from build123d import *

# Parameters (mm, degrees)
SKETCH1_W           = 304.8
SKETCH1_H           = 89.8
SKETCH1_R           = 14.2875
SKETCH1_R_2         = 2.54
SKETCH1_R_3         = 17.145
BOSS_EXTRUDE1_DEPTH = 6.35
SKETCH2_W           = 114.9
SKETCH2_H           = 89.8
SKETCH2_R           = 2.54
SKETCH2_R_2         = 17.145
CUT_EXTRUDE1_DEPTH  = 10
SKETCH4_R           = 6.35
SKETCH4_R_2         = 1.778
BOSS_EXTRUDE2_DEPTH = 6.35
FILLET1_R           = 10
FILLET2_R           = 7.5
SKETCH7_R           = 2.05
CUT_EXTRUDE2_DEPTH  = 10
SCALE1_SCALE        = 0.333333333


with BuildPart() as part:
    # Sketch1 → Boss-Extrude1 (new body)
    with BuildSketch(Plane.XY):
        with Locations((152.4, 44.9)):
            Rectangle(SKETCH1_W, SKETCH1_H)
        with Locations((152.4, 44.9)):
            Circle(SKETCH1_R, mode=Mode.SUBTRACT)
        with Locations((109.401585406, 62.859439014)):
            Circle(SKETCH1_R_2, mode=Mode.SUBTRACT)
        with Locations((109.399439014, 26.938414594)):
            Circle(SKETCH1_R_2, mode=Mode.SUBTRACT)
        with Locations((73.478414594, 26.940560986)):
            Circle(SKETCH1_R_2, mode=Mode.SUBTRACT)
        with Locations((73.480560986, 62.861585406)):
            Circle(SKETCH1_R_2, mode=Mode.SUBTRACT)
        with Locations((91.44, 44.9)):
            Circle(SKETCH1_R_3, mode=Mode.SUBTRACT)
        with Locations((195.400560986, 62.861585406)):
            Circle(SKETCH1_R_2, mode=Mode.SUBTRACT)
        with Locations((231.321585406, 62.859439014)):
            Circle(SKETCH1_R_2, mode=Mode.SUBTRACT)
        with Locations((231.319439014, 26.938414594)):
            Circle(SKETCH1_R_2, mode=Mode.SUBTRACT)
        with Locations((195.398414594, 26.940560986)):
            Circle(SKETCH1_R_2, mode=Mode.SUBTRACT)
        with Locations((213.36, 44.9)):
            Circle(SKETCH1_R_3, mode=Mode.SUBTRACT)
    extrude(amount=BOSS_EXTRUDE1_DEPTH)

    # Sketch2 → Cut-Extrude1 (cut)
    with BuildSketch(Plane.XY.offset(6.35)):
        with Locations((247.35, 44.9)):
            Rectangle(SKETCH2_W, SKETCH2_H)
        with Locations((195.398414594, 26.940560986)):
            Circle(SKETCH2_R, mode=Mode.SUBTRACT)
        with Locations((231.319439014, 26.938414594)):
            Circle(SKETCH2_R, mode=Mode.SUBTRACT)
        with Locations((213.36, 44.9)):
            Circle(SKETCH2_R_2, mode=Mode.SUBTRACT)
        with Locations((195.400560986, 62.861585406)):
            Circle(SKETCH2_R, mode=Mode.SUBTRACT)
        with Locations((231.321585406, 62.859439014)):
            Circle(SKETCH2_R, mode=Mode.SUBTRACT)
        with Locations((57.45, 44.9)):
            Rectangle(SKETCH2_W, SKETCH2_H)
        with Locations((73.478414594, 26.940560986)):
            Circle(SKETCH2_R, mode=Mode.SUBTRACT)
        with Locations((109.399439014, 26.938414594)):
            Circle(SKETCH2_R, mode=Mode.SUBTRACT)
        with Locations((91.44, 44.9)):
            Circle(SKETCH2_R_2, mode=Mode.SUBTRACT)
        with Locations((73.480560986, 62.861585406)):
            Circle(SKETCH2_R, mode=Mode.SUBTRACT)
        with Locations((109.401585406, 62.859439014)):
            Circle(SKETCH2_R, mode=Mode.SUBTRACT)
    extrude(amount=-CUT_EXTRUDE1_DEPTH, mode=Mode.SUBTRACT)

    # Sketch4 → Boss-Extrude2 (add)
    with BuildSketch(Plane.XY.offset(6.35)):
        with BuildLine():
            Line((189.9, 0), (154.512001483, -31.80682216))
            ThreePointArc((154.512001483, -31.80682216), (141.221457874, -35.647397134), (129.96508312, -27.604848226))
            Line((129.96508312, -27.604848226), (114.9, 0))
            Line((114.9, 0), (189.9, 0))
        make_face()
        with Locations((143.9, -20)):
            Circle(SKETCH4_R, mode=Mode.SUBTRACT)
        with Locations((143.9, -29.779)):
            Circle(SKETCH4_R_2, mode=Mode.SUBTRACT)
        with Locations((134.121, -20)):
            Circle(SKETCH4_R_2, mode=Mode.SUBTRACT)
        with Locations((153.679, -20)):
            Circle(SKETCH4_R_2, mode=Mode.SUBTRACT)
        with Locations((143.9, -10.221)):
            Circle(SKETCH4_R_2, mode=Mode.SUBTRACT)
    extrude(amount=-BOSS_EXTRUDE2_DEPTH)

    # Fillet1
    fillet1_edges = [part.edges().sort_by_distance(p)[0] for p in [
        (189.9, 0, 3.175),
        (114.9, 0, 3.175),
    ]]
    fillet(fillet1_edges, radius=FILLET1_R)

    # Fillet2
    fillet2_edges = [part.edges().sort_by_distance(p)[0] for p in [
        (114.9, 89.8, 3.175),
        (189.9, 89.8, 3.175),
    ]]
    fillet(fillet2_edges, radius=FILLET2_R)

    # Sketch7 → Cut-Extrude2 (cut)
    with BuildSketch(Plane.XY.offset(6.35)):
        with Locations((179.9, 69.8)):
            Circle(SKETCH7_R)
        with Locations((124.9, 69.8)):
            Circle(SKETCH7_R)
        with Locations((124.9, 20)):
            Circle(SKETCH7_R)
        with Locations((179.9, 20)):
            Circle(SKETCH7_R)
    extrude(amount=-CUT_EXTRUDE2_DEPTH, mode=Mode.SUBTRACT)


with BuildPart() as part_1:
    # Scale1: scaled about (151.749134019, 33.595748841, 3.175)
    add(part.part.scale(SCALE1_SCALE).moved(Location((101.166089346, 22.397165894, 2.116666667))))


solid = part_1.part
Can you work these out from the model? Positions are in its coordinate system, mm. Give positions to 0.01 mm unless a question says otherwise; leave off trailing zeros. Loops run counter-clockwise (first coordinate to the right, second up) from the corner with the lowest first, then second, coordinate; pieces in that order, holes last. Notation, with made-up numbers: (3, -22) -> (52, -22) arc R17 cw to (52, -8) -> close; hole circle Ø3 at (-10, 37.5). An arc over 180 degrees is marked (long way). Return JSON: item names as keys, results as strings.
Q1. I need wall thicknesses on probe 1 along Y at (x, z) = (151, 3.9); probe 2 along Y at (x, z) = (147.75, 3.45); probe 3 along X at (y, z) = (15.5, 3.8). Which ranges of each line are inside material? Lowest first, please.
Checks:
{"probe 1": "y = 10.78 to 14.73, 16.73 to 32.7, 42.03 to 52.33", "probe 2": "y = 10.62 to 14.13, 17.33 to 35.15, 39.58 to 52.33", "probe 3": "x = 143.23 to 145.33, 146.42 to 147.03, 151.24 to 151.85, 152.94 to 156.79"}
Q2. We'd pull the mould along X, two halves only. Please class faces 1 (the face through (149.45, 19.49, 3.19)), 2 (the face through (152, 52.33, 3)), 3 (the face through (139.466, 36, 3)): released by +X, released by -X, zero draft, split by the parting line, or undercut.
Checks:
{"face 1": "undercut", "face 2": "zero draft", "face 3": "released by -X"}
Q3. I want a section at C-C, the plane z = 2.8. Count the separate pieces of the cut face and the enclosed holes in it, then the cut area to 3 significant figures.
Checks:
{"separate pieces": "1", "enclosed holes": "10", "area": "828 mm2"}
Q4. I want a section at A-A, the plane x = 161. List the corners of the cut face in (y, z) for me, then the cut area to 3 significant figures.
Checks:
{"outline": "(19.28, 2.12) -> (28.39, 2.12) -> (28.39, 4.23) -> (19.28, 4.23) -> close; (29.73, 2.12) -> (44.99, 2.12) -> (44.99, 4.23) -> (29.73, 4.23) -> close; (46.33, 2.12) -> (52.33, 2.12) -> (52.33, 4.23) -> (46.33, 4.23) -> close", "area": "64.3 mm2"}
Q5. I want a section at D-D, the plane x = 142.75. List the corners of the cut face in (y, z) for me, then the cut area to 3 significant figures.
Checks:
{"outline": "(16.38, 2.12) -> (28.38, 2.12) -> (28.38, 4.23) -> (16.38, 4.23) -> close; (29.75, 2.12) -> (44.98, 2.12) -> (44.98, 4.23) -> (29.75, 4.23) -> close; (46.35, 2.12) -> (52.33, 2.12) -> (52.33, 4.23) -> (46.35, 4.23) -> close", "area": "70.3 mm2"}
Q6. I want a section at B-B, the plane y = 39. List the corners of the cut face in (x, z) for me, then the cut area to 3 significant figures.
Checks:
{"outline": "(139.47, 2.12) -> (147.49, 2.12) -> (147.49, 4.23) -> (139.47, 4.23) -> close; (156.44, 2.12) -> (164.47, 2.12) -> (164.47, 4.23) -> (156.44, 4.23) -> close", "area": "34.0 mm2"}
